Source: CAD feature listing. Evaluate the final solid. Frame: model axes, mm. A direction names the side the tool comes from. Round coordinates to 2 decimals unless told otherwise and drop trailing zeros. Loops run counter-clockwise (first coordinate to the right, second up) from the corner with the lowest first, then second, coordinate; pieces in that order, holes last.
Item 1: Section query D-D on z = 33. Return loops of the section in (x, y).
Item 2: Section query A-A on x = 5. Return loops of the section in (y, z).
Item 3: Ray query, L1, parallel to Z at x = 14.5, y = 75; L2, parallel to X at y = -25.5, z = -7.5; L3, parallel to Z at x = 39, y = -164. Return the intervals inside material, ascending.
Item 4: First-contact query: P1, Ø1.5, axis at x = -17, y = -165.5, coming from the +Z side; P2, Ø4, axis at x = 35, y = 142, coming from the -Z side; P3, Ø6, axis at x = -42, y = 193, coming from the -Z side. Flat tips, straight axial feed; report the tip coordinate or a pass-through.
Item 5: Section query C-C on z = 7. Return loops of the section in (x, y).
Item 6: Section query B-B on y = -95.5. Give the number of separate pieces and of enclosed holes in the cut face, then the cut area to 3 significant figures.
Item 7: Pull-direction query (Z, two-part tool) for faces 1 (the flat face through (-20.394, -3, -10)), 2 (the flat face through (-15, 255, 63)), 3 (the flat face through (-49, -8.8, -15.3)), 4 (the flat face through (35, -3, 1.3)); classes: released by +Z, released by -Z, zero draft, split by the parting line, or undercut.
Item 8: Access query for faces 5 (the flat face through (-4, 250, -3)), 6 (the flat face through (0, 59, -3.75)), 7 (the flat face through (0, 4, 0)). Directions: +Z, -Z, +X, -X, +Y, -Y. A direction counts if a zero-diameter tool reaches every point of the face in a straight line with its end or side. Return the directions, or none.
```python
from build123d import *

# Parameters (mm, degrees)
F1_DEPTH       = 250
F2_W           = 38
F2_H           = 13
F3_DEPTH       = 250
F4_T1_DEPTH    = 509.3674969976
F5_R           = 9
F6_R           = 2
F8_DEPTH       = 764
F8_DEPTH_BACK  = 500.001
F10_DEPTH      = 22.2193051812
F10_DEPTH_BACK = 1.301
F12_DEPTH      = 1.3010001
F12_DEPTH_BACK = 22.219305294
F13_T1_DEPTH   = 3.7499991487
F13_T6_DEPTH   = 15.0134832828
F13_S7_R       = 200
F13_T8_DEPTH   = 10
F13_T12_DEPTH  = 15.0134832828
F13_S13_R      = 200
F13_T14_DEPTH  = 10
F13_T15_DEPTH  = 28.7499991487
F13_T17_DEPTH  = 27.5134832828
F15_DEPTH      = 15
F16_R          = 27.5
F17_DEPTH      = 100
F19_D          = 40


# Not quite as in the source:
# - a fillet or chamfer that OpenCascade refuses, or shapes differently, is made with other operations: its cross-section is extruded or revolved along the edge and cut away or added
# - an extrude ends at something that could not be found from the text; its depth is read off the source's solid


with BuildPart() as f1:
    # F0 (on Front) → F1 (new body, symmetric)
    with BuildSketch(Plane.XZ):
        with BuildLine():
            Line((22.5, 0), (0, 0))
            Line((0, 0), (-22.5, 0))
            Line((-22.5, 0), (-22.5, 1.3))
            Line((-22.5, 1.3), (-49.1090036882, 1.3))
            Line((-49.1090036882, 1.3), (-57.5, -8.7))
            Line((-57.5, -8.7), (-57.5, -12.7))
            Line((-57.5, -12.7), (-40.1794919243, -22.7))
            ThreePointArc((-40.1794919243, -22.7), (0, -18.6224551416), (40.1794919243, -22.7))
            Line((40.1794919243, -22.7), (57.5, -12.7))
            Line((57.5, -12.7), (57.5, -8.7))
            Line((57.5, -8.7), (49.1090036882, 1.3))
            Line((49.1090036882, 1.3), (22.5, 1.3))
            Line((22.5, 1.3), (22.5, 0))
        make_face()
    extrude(amount=F1_DEPTH, both=True)

    # F2 (on Front) → F3 (cut, symmetric)
    with BuildSketch(Plane.XZ):
        with Locations((0, -10.2499991487)):
            Rectangle(F2_W, F2_H)
    extrude(amount=F3_DEPTH, both=True, mode=Mode.SUBTRACT)

    # F4: fillet of radius 2 on 2 edges, made by hand

    # F4_s2 → F4_t1 (cut)
    with BuildSketch(Plane.XZ.offset(-254.6837484988)):
        with BuildLine():
            ThreePointArc((24.3734993995, 1.3), (23.2333239744, 0.9431676725), (22.5, 0))
            Line((22.5, 0), (22.5, 1.3))
            Line((22.5, 1.3), (24.3734993995, 1.3))
        make_face()
        with BuildLine():
            ThreePointArc((-24.3734993995, 1.3), (-23.2333239744, 0.9431676725), (-22.5, 0))
            Line((-22.5, 0), (-22.5, 1.3))
            Line((-22.5, 1.3), (-24.3734993995, 1.3))
        make_face()
    extrude(amount=F4_T1_DEPTH, mode=Mode.SUBTRACT)

    # F5
    f5_edges = [f1.edges().sort_by_distance(p)[0] for p in [
        (-49.109004, 0, 1.3),
        (49.109004, 0, 1.3),
        (40.179492, 0, -22.7),
        (-40.179492, 0, -22.7),
    ]]
    fillet(f5_edges, radius=F5_R)

    # F6
    f6_edges = [f1.edges().sort_by_distance(p)[0] for p in [
        (-57.5, 0, -8.7),
        (-57.5, 0, -12.7),
        (57.5, 0, -8.7),
        (57.5, 0, -12.7),
    ]]
    fillet(f6_edges, radius=F6_R)

    # F7 (on face) → F8 (cut, two sides)
    with BuildSketch(Plane.XZ.offset(250)) as f8_sk:
        with BuildLine():
            ThreePointArc((-37.3093701274, -20.0978700124), (-28.8776819579, -18.697270423), (-20.3942914958, -17.6546147432))
            Line((-20.3942914958, -17.6546147432), (-20.3942914958, -2.4123612095))
            Line((-20.3942914958, -2.4123612095), (-22.3942914958, -2.4123612095))
            ThreePointArc((-22.3942914958, -2.4123612095), (-23.0649271969, -1.1875057717), (-24.3734993995, -0.7))
            Line((-24.3734993995, -0.7), (-44.9122347648, -0.7))
            ThreePointArc((-44.9122347648, -0.7), (-47.870562597, -1.3558454907), (-50.2745458667, -3.2004867322))
            Line((-50.2745458667, -3.2004867322), (-55.9308095341, -9.9413592785))
            ThreePointArc((-55.9308095341, -9.9413592785), (-56.149572844, -10.7577950659), (-55.664765091, -11.450172292))
            Line((-55.664765091, -11.450172292), (-42.1022690923, -19.2804830077))
            ThreePointArc((-42.1022690923, -19.2804830077), (-39.7790673433, -20.1186780608), (-37.3093701274, -20.0978700124))
        make_face()
        with BuildLine():
            Line((22.3942914958, -2.4123612095), (20.3942914958, -2.4123612095))
            Line((20.3942914958, -2.4123612095), (20.3942914958, -17.6546147432))
            ThreePointArc((20.3942914958, -17.6546147432), (28.8776819579, -18.697270423), (37.3093701274, -20.0978700124))
            ThreePointArc((37.3093701274, -20.0978700124), (39.7790673433, -20.1186780608), (42.1022690923, -19.2804830077))
            Line((42.1022690923, -19.2804830077), (55.664765091, -11.450172292))
            ThreePointArc((55.664765091, -11.450172292), (56.149572844, -10.7577950659), (55.9308095341, -9.9413592785))
            Line((55.9308095341, -9.9413592785), (50.2745458667, -3.2004867322))
            ThreePointArc((50.2745458667, -3.2004867322), (47.870562597, -1.3558454907), (44.9122347648, -0.7))
            Line((44.9122347648, -0.7), (24.3734993995, -0.7))
            ThreePointArc((24.3734993995, -0.7), (23.0649271969, -1.1875057717), (22.3942914958, -2.4123612095))
        make_face()
    extrude(amount=F8_DEPTH, mode=Mode.SUBTRACT)
    extrude(f8_sk.sketch, amount=-F8_DEPTH_BACK, mode=Mode.SUBTRACT)

    # F9 (on Top) → F10 (cut, two sides)
    with BuildSketch(Plane.XY) as f10_sk:
        with BuildLine():
            ThreePointArc((-57.5, 200), (0, 257.5), (57.5, 200))
            Line((57.5, 200), (57.5, 280))
            Line((57.5, 280), (-57.5, 280))
            Line((-57.5, 280), (-57.5, 200))
        make_face()
    extrude(amount=-F10_DEPTH, mode=Mode.SUBTRACT)
    extrude(f10_sk.sketch, amount=F10_DEPTH_BACK, mode=Mode.SUBTRACT)

    # F11 (on Top) → F12 (cut, two sides)
    with BuildSketch(Plane.XY) as f12_sk:
        Polygon((-43.2975540478, -250), (-68, -216), (-68, -346), (68, -346), (68, -216), (43.2975540478, -250), (16, -250), (16, -140), (-16, -140), (-16, -250), align=None)
    extrude(amount=F12_DEPTH, mode=Mode.SUBTRACT)
    extrude(f12_sk.sketch, amount=-F12_DEPTH_BACK, mode=Mode.SUBTRACT)

    # F13: fillet of radius 5 on 8 edges, made by hand

    # F13_s2 → F13_t1 (join)
    with BuildSketch(Plane.XY.offset(-3.7499991487)):
        with BuildLine():
            ThreePointArc((-11, -140), (-14.5355339059, -141.4644660941), (-16, -145))
            Line((-16, -145), (-16, -140))
            Line((-16, -140), (-11, -140))
        make_face()
        with BuildLine():
            ThreePointArc((16, -145), (14.5355339059, -141.4644660941), (11, -140))
            Line((11, -140), (16, -140))
            Line((16, -140), (16, -145))
        make_face()
    extrude(amount=F13_T1_DEPTH)


with BuildPart() as f13_tool4:
    # F13_s5 → F13_t6 (new body)
    with BuildSketch(Plane.XY.offset(-16.7499991487)):
        with BuildLine():
            ThreePointArc((-16, -145), (-14.5355339059, -141.4644660941), (-11, -140))
            Line((-11, -140), (-16, -140))
            Line((-16, -140), (-16, -145))
        make_face()
    extrude(amount=-F13_T6_DEPTH)

    # F13_s7 → F13_t8 (cut, symmetric)
    with BuildSketch(Plane.XZ.offset(142.5)):
        with Locations((0, -218.6224551416)):
            Circle(F13_S7_R)
    extrude(amount=F13_T8_DEPTH, both=True, mode=Mode.SUBTRACT)


with BuildPart() as f1_1:
    add(f1.part)

    # F13_t3: union F13_tool4
    add(f13_tool4.part)


with BuildPart() as f13_tool10:
    # F13_s11 → F13_t12 (new body)
    with BuildSketch(Plane.XY.offset(-31.7634824315)):
        with BuildLine():
            ThreePointArc((16, -145), (14.5355339059, -141.4644660941), (11, -140))
            Line((11, -140), (16, -140))
            Line((16, -140), (16, -145))
        make_face()
    extrude(amount=F13_T12_DEPTH)

    # F13_s13 → F13_t14 (cut, symmetric)
    with BuildSketch(Plane.XZ.offset(142.5)):
        with Locations((0, -218.6224551416)):
            Circle(F13_S13_R)
    extrude(amount=F13_T14_DEPTH, both=True, mode=Mode.SUBTRACT)


with BuildPart() as f1_2:
    add(f1_1.part)

    # F13_t9: union F13_tool10
    add(f13_tool10.part)

    # F13_s16 → F13_t15 (cut)
    with BuildSketch(Plane.XY.offset(-16.2499991487)):
        with BuildLine():
            ThreePointArc((21, -250), (17.4644660941, -248.5355339059), (16, -245))
            Line((16, -245), (16, -250))
            Line((16, -250), (21, -250))
        make_face()
        with BuildLine():
            ThreePointArc((-21, -250), (-17.4644660941, -248.5355339059), (-16, -245))
            Line((-16, -245), (-16, -250))
            Line((-16, -250), (-21, -250))
        make_face()
    extrude(amount=F13_T15_DEPTH, mode=Mode.SUBTRACT)

    # F13_s18 → F13_t17 (cut)
    with BuildSketch(Plane.XY.offset(-31.7634824315)):
        with BuildLine():
            ThreePointArc((21, -250), (17.4644660941, -248.5355339059), (16, -245))
            Line((16, -245), (16, -250))
            Line((16, -250), (21, -250))
        make_face()
        with BuildLine():
            ThreePointArc((-21, -250), (-17.4644660941, -248.5355339059), (-16, -245))
            Line((-16, -245), (-16, -250))
            Line((-16, -250), (-21, -250))
        make_face()
    extrude(amount=F13_T17_DEPTH, mode=Mode.SUBTRACT)

    # F14 (on Right) → F15 (join, symmetric)
    with BuildSketch(Plane.YZ):
        with BuildLine():
            ThreePointArc((297.3819995028, 160), (245.9666940414, 74.662277853), (180, 0))
            Line((180, 0), (250, 0))
            ThreePointArc((250, 0), (267.6550746197, 46.4758946867), (311.7145367693, 69.5079211245))
            Line((311.7145367693, 69.5079211245), (313.0254460068, 61.2311659405))
            Line((313.0254460068, 61.2311659405), (358.4591096742, 68.4271513323))
            Line((358.4591096742, 68.4271513323), (342.8156631702, 167.1959853919))
            Line((342.8156631702, 167.1959853919), (297.3819995028, 160))
        make_face()
    extrude(amount=F15_DEPTH, both=True)

    # F16 (on face) → F17 (join, through all)
    with BuildSketch(Plane(origin=(0, -17.4439040266, 110.1364754698), x_dir=(1, 0, 0), z_dir=(0, -0.156434465, 0.9876883406))):
        with Locations((0, 341.7502480182)):
            Circle(F16_R)
    extrude(amount=-F17_DEPTH)

    # F19 (through all)
    with Locations(Plane(origin=(0, -17.4439040266, 110.1364754698), x_dir=(1, 0, 0), z_dir=(0, -0.156434465, 0.9876883406))):
        with Locations((0, 341.7502480182)):
            Hole(F19_D / 2)


solid = f1_2.part
```
Data:
1. outline: (-15, 212.16) - (15, 212.16) - (15, 258.27) - (-15, 258.27) - close
2. outline: (-140, -18.68) - (250, -18.68) - (250, -16.75) - (-140, -16.75) - close; (-140, -3.75) - (250, -3.75) - (250, 0) arc R70 cw to (307.72, 68.91) - (309.03, 60.6) - (316.62, 61.8) - (300.97, 160.57) - (293.39, 159.37) - (294.29, 153.72) arc R550 cw to (180, 0) - (-140, 0) - close; (339.23, 166.63) - (354.87, 67.86) - (362.45, 69.06) - (346.81, 167.83) - close
3. L1: z = -19.15 to -16.75, -3.75 to 0
3. L2: x = -56.49 to -53.88, -20.39 to -19, 19 to 20.39, 53.88 to 56.49
3. L3: z = -22.21 to -20.21, -0.7 to 1.3
4. P1: stops at z = 0
4. P2: stops at z = -22.07
4. P3: stops at z = -22.21
5. outline: (-15, 187.28) - (15, 187.28) - (15, 250.35) - (-15, 250.35) - close
6. separate pieces: 1
6. enclosed holes: 3
6. area: 606 mm2
7. face 1: undercut
7. face 2: zero draft
7. face 3: undercut
7. face 4: released by +Z
8. face 5: -Z, +X, -X, +Y
8. face 6: +Y, -Y
8. face 7: +Z, -Y
